Input: part model. Units: mm. Frame: model coordinates. A direction names the side the tool comes from. Give positions to 0.01 mm unless a question says otherwise; leave off trailing zeros. Loops run counter-clockwise (first coordinate to the right, second up) from the corner with the lowest first, then second, coordinate; pieces in that order, holes last. Notation, with made-up numbers: (17, 34.5) - (52, 34.5) arc R21 cw to (52, 61.5) - close; hole circle Ø4 at (67.5, 31). An arc over 180 degrees is marked (long way). Answer as a JSON object with one key per item and string values. Group by question number.
(1) Section query D-D (z = -30). Return loops of the section in (x, y).
(2) Pin query (flat end, axial travel): P1, Ø1.9, axis at x = -54, y = -3, coming from the -Z side; P2, Ø1.9, axis at x = -40.5, y = -2, coming from the +Z side; P3, Ø1.5, axis at x = 23, z = -6.5, coming from the +Y side; P4, Ø1.9, axis at y = -2.5, z = 33, coming from the -X side. Return the tip coordinate at first contact, or that it passes through.
(3) Material intervals for L1, parallel to Z at x = -51, y = -1.5; L2, parallel to Z at x = 1, y = -6; L3, parallel to X at y = -0.75, z = 6, sorted ascending.
(4) Section query B-B (x = 11). Return loops of the section in (y, z), plus the area to 3 significant figures.
(5) Mould query, pull axis Z, two halves, no side actions, for faces 1 (the flat face through (6, -3, 38.1)), 2 (the flat face through (38.1, -3, 1)), 3 (the flat face through (-54, -3, -22.86)), 4 (the flat face through (-16.075, -3.131, -9.319)). Classes: +Z half, -Z half, draft (parallel to the pull), parting line (faces both ways), or undercut.
(6) Section query C-C (x = -31.5). Return loops of the section in (y, z).
(7) Section query A-A (z = -5). Return loops of the section in (x, y).
(8) Access query for faces 5 (the flat face through (-48, -3, 10.16)), 6 (the flat face through (0, -3, 18.581)), 7 (the flat face through (-25.4, -3, -31)), 8 (the flat face through (-46.203, -3, -22)). Directions: +Z, -Z, +X, -X, +Y, -Y. A direction counts if a zero-diameter tool reaches every point of the face in a straight line with its end or side. Return the directions, or none.
```python
from build123d import *

# Parameters (mm, degrees)
BOSS_EXTRUDE1_DEPTH = 6.35


with BuildPart() as part:
    # Sketch1 → Boss-Extrude1 (new body)
    with BuildSketch(Plane(origin=(0, 0, 0), x_dir=(1, 0, 0), z_dir=(0, 1, 0))):
        Polygon((-25.4, -38.1), (38.1, -38.1), (38.1, 38.1), (-25.4, 38.1), (-25.4, 22.86), (-38.1, 22.86), (-46.2026, 22.86), (-46.2026, 20.447), (-44.0944, 20.447), (-44.0944, 17.78), (-51.9684, 17.78), (-51.9684, 20.447), (-49.8602, 20.447), (-49.8602, 22.86), (-57.9628, 22.86), (-57.9628, 10.16), (-38.1, 10.16), (-38.1, -10.16), (-57.9628, -10.16), (-57.9628, -22.86), (-49.8602, -22.86), (-49.8602, -20.447), (-51.9684, -20.447), (-51.9684, -17.78), (-44.0944, -17.78), (-44.0944, -20.447), (-46.2026, -20.447), (-46.2026, -22.86), (-38.1, -22.86), (-25.4, -22.86), align=None)
        Polygon((-2.389310714, -18.580574179), (2.389310714, -18.580574179), (14.896593899, -11.359490865), (17.285904613, -7.221083314), (17.285904613, 7.221083314), (14.896593899, 11.359490865), (2.389310714, 18.580574179), (-2.389310714, 18.580574179), (-14.896593899, 11.359490865), (-17.285904613, 7.221083314), (-17.285904613, -7.221083314), (-14.896593899, -11.359490865), align=None, mode=Mode.SUBTRACT)
    extrude(amount=-BOSS_EXTRUDE1_DEPTH)


solid = part.part
```
Recorded:
{
 "1": {"outline": "(-25.4, -6.35) - (38.1, -6.35) - (38.1, 0) - (-25.4, 0) - close"},
 "2": {"P1": "stops at z = -22.86", "P2": "stops at z = 22.86", "P3": "stops at y = 0", "P4": "stops at x = -25.4"},
 "3": {"L1": "z = -22.86 to -20.45, -17.78 to -10.16, 10.16 to 17.78, 20.45 to 22.86", "L2": "z = -38.1 to -18.58, 18.58 to 38.1", "L3": "x = -38.1 to -17.29, 17.29 to 38.1"},
 "4": {"outline": "(-6.35, -38.1) - (0, -38.1) - (0, -13.61) - (-6.35, -13.61) - close; (-6.35, 13.61) - (0, 13.61) - (0, 38.1) - (-6.35, 38.1) - close", "area": "311 mm^2"},
 "5": {"face 1": "+Z half", "face 2": "draft", "face 3": "-Z half", "face 4": "undercut"},
 "6": {"outline": "(-6.35, -22.86) - (0, -22.86) - (0, 22.86) - (-6.35, 22.86) - close"},
 "7": {"outline": "(-38.1, -6.35) - (-17.29, -6.35) - (-17.29, 0) - (-38.1, 0) - close; (17.29, -6.35) - (38.1, -6.35) - (38.1, 0) - (17.29, 0) - close"},
 "8": {"face 5": "-X, +Y, -Y", "face 6": "+Y, -Y", "face 7": "-Z, -X, +Y, -Y", "face 8": "-Z, +Y, -Y"}
}
